Design review of the part built by this model. Coordinates are the model's own, in mm. Face numbers are marked on the shaded views. A direction names the side the tool comes from. Give positions to 0.01 mm unless a question says otherwise; leave off trailing zeros. Write each loop counter-clockwise with the first axis right and the second up, starting at its lowest first coordinate (ties: lowest second). Pieces come first, ordered by that corner, then holes. Notation, with made-up numbers: M 34,89 L 39,89 A26 ccw 39,109 Z; hole C 19.5,14.25 d7. An arc over 180 degrees is marked long. Use one line per item in the form item = value. Start each with the question number.
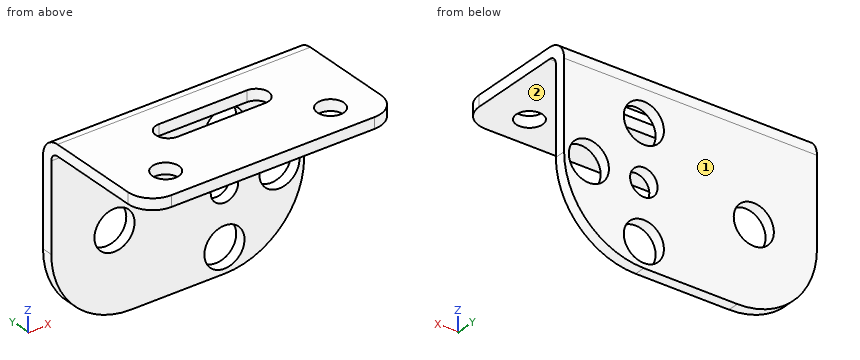
from build123d import *

# Parameters (mm, degrees)
SKETCH_3_W          = 46
SKETCH_3_H          = 33.8
EXTRUDE_1_DEPTH     = 2
FILLET_1_R          = 14.5
SKETCH_4_R          = 2.5
SKETCH_4_R_2        = 3.65
CUT_EXTRUDE_1_DEPTH = 2
SKETCH_5_W          = 46
SKETCH_5_H          = 2
EXTRUDE_2_DEPTH     = 23
FILLET_2_R          = 4.5
FILLET_3_R          = 3.5
FILLET_4_R          = 1.5
SKETCH_6_R          = 2.4
CUT_EXTRUDE_2_DEPTH = 25


with BuildPart() as part:
    # 草图3 → 凸台-拉伸1 (new body)
    with BuildSketch(Plane(origin=(0, 0, 0), x_dir=(1, 0, 0), z_dir=(0, 1, 0))):
        with Locations((23, 16.9)):
            Rectangle(SKETCH_3_W, SKETCH_3_H)
    extrude(amount=EXTRUDE_1_DEPTH)

    # 圆角1
    fillet_1_edges = [part.edges().sort_by_distance(p)[0] for p in [
        (0, 1, -33.8),
        (46, 1, -33.8),
    ]]
    fillet(fillet_1_edges, radius=FILLET_1_R)

    # 草图4 → 切除-拉伸1 (cut)
    with BuildSketch(Plane(origin=(0, 2, 0), x_dir=(1, 0, 0), z_dir=(0, 1, 0))):
        with Locations(Location((31.5, 19.3, 0), (0, 0, 270))):
            Circle(SKETCH_4_R)
        with Locations(Location((41.5, 19.3, 0), (0, 0, 270))):
            Circle(SKETCH_4_R_2)
        with Locations(Location((31.5, 29.3, 0), (0, 0, 270))):
            Circle(SKETCH_4_R_2)
        with Locations(Location((31.5, 9.3, 0), (0, 0, 270))):
            Circle(SKETCH_4_R_2)
        with Locations(Location((11.5, 19.3, 0), (0, 0, 270))):
            Circle(SKETCH_4_R_2)
    extrude(amount=-CUT_EXTRUDE_1_DEPTH, mode=Mode.SUBTRACT)

    # 草图5 → 凸台-拉伸2 (add)
    with BuildSketch(Plane.XZ):
        with Locations((23, -1)):
            Rectangle(SKETCH_5_W, SKETCH_5_H)
    extrude(amount=EXTRUDE_2_DEPTH)

    # 圆角2
    fillet_2_edges = [part.edges().sort_by_distance(p)[0] for p in [
        (0, -23, -1),
        (46, -23, -1),
    ]]
    fillet(fillet_2_edges, radius=FILLET_2_R)

    # 圆角3
    fillet_3_edges = [part.edges().sort_by_distance(p)[0] for p in [
        (23, 2, 0),
    ]]
    fillet(fillet_3_edges, radius=FILLET_3_R)

    # 圆角4
    fillet_4_edges = [part.edges().sort_by_distance(p)[0] for p in [
        (23, 0, -2),
    ]]
    fillet(fillet_4_edges, radius=FILLET_4_R)

    # 草图6 → 切除-拉伸2 (cut)
    with BuildSketch(Plane.XY):
        with Locations((8, -17)):
            Circle(SKETCH_6_R)
        with Locations((38, -17)):
            Circle(SKETCH_6_R)
        with BuildLine():
            Line((15.25, -5.75), (31.25, -5.75))
            ThreePointArc((31.25, -5.75), (33.5, -8), (31.25, -10.25))
            Line((31.25, -10.25), (15.25, -10.25))
            ThreePointArc((15.25, -10.25), (13, -8), (15.25, -5.75))
        make_face()
    extrude(amount=-CUT_EXTRUDE_2_DEPTH, mode=Mode.SUBTRACT)


solid = part.part
1. We need section A-A (z = -27). State the section outline as (x, y) points, and give its area (3 significant figures).
2. To check wall thickness, follow L1, parallel to Y at x = 9, z = -4; L2, parallel to Y at x = 8, z = -1.05; L3, parallel to Z at x = 34, y = -6. State the ranges of each line that lie inside material, in increasing order.
3. Clearance check with flat-ended pins moving along their axes: pin 1 Ø8.5 at (x, z) = (41.5, -19.3) entering from -Y; pin 2 Ø3 at (x, y) = (39, -15.5) entering from -Z; pin 3 Ø1 at (y, z) = (-2, -14) entering from -X; pin 4 Ø5 at (x, z) = (27, -5.5) entering from -Y. State where each tip first meets the part, or that it passes through.
4. For the marked faces 1 and 2, list the 3-axis set-ups (+Z, -Z, +X, -X, +Y, -Y) from which the entire face can be reached by the end or side of a thin tool; tool diameter is ignored.
5. We need section B-B (y = -8). State the section outline as (x, z) points, and give its area (3 significant figures).
6. We need section C-C (y = -17). State the section outline as (x, z) points.
7. We need section D-D (x = 37). State the section outline as (y, z) points.
Answer block:
q1.outline = M 2.21,0 L 28.67,0 L 28.67,2 L 2.21,2 Z; M 34.33,0 L 43.79,0 L 43.79,2 L 34.33,2 Z
q1.area = 71.8 mm^2
q2.L1 = 0 to 2
q2.L2 = -23 to -19.4, -14.6 to 1
q2.L3 = -2 to 0
q3.pin_1 = 0
q3.pin_2 = -2
q3.pin_3 = through
q3.pin_4 = -0.09
q4.face_1 = +Z, -Z, +X, -X, +Y
q4.face_2 = -Z, +X, -X, -Y
q5.outline = M 0,-2 L 13,-2 L 13,0 L 0,0 Z; M 33.5,-2 L 46,-2 L 46,0 L 33.5,0 Z
q5.area = 51.0 mm^2
q6.outline = M 0,-2 L 5.6,-2 L 5.6,0 L 0,0 Z; M 10.4,-2 L 35.6,-2 L 35.6,0 L 10.4,0 Z; M 40.4,-2 L 46,-2 L 46,0 L 40.4,0 Z
q7.outline = M -23,-2 L -19.18,-2 L -19.18,0 L -23,0 Z; M -14.82,-2 L -1.5,-2 A1.5 cw 0,-3.5 L 0,-32.72 L 2,-32.72 L 2,-3.5 A3.5 ccw -1.5,0 L -14.82,0 Z
